```python
from build123d import *

# Parameters (mm, degrees)
SKETCH1_W = 17.5
SKETCH1_H = 8
FILLET1_R = 1


with BuildPart() as part:
    # Sketch1 → Revolve1 (revolve)
    with BuildSketch(Plane.XY, mode=Mode.PRIVATE) as revolve1_sk:
        with Locations((8.75, 4)):
            Rectangle(SKETCH1_W, SKETCH1_H)
    revolve(revolve1_sk.sketch.rotate(Axis((0, 0, 0), (0, 1, 0)), 90), axis=Axis((0, 0, 0), (0, 1, 0)))

    # Sketch2 → CSK for M3 Countersunk Flat Head Screw1 (revolve, cut)
    with BuildSketch(Plane(origin=(0, 8, 0), x_dir=(0, 0, 1), z_dir=(1, 0, 0))):
        Polygon((0, 0), (0, 8), (7.25, 8), (7.25, 5.25), (12.5, 0), align=None)
    revolve(axis=Axis((0, 14.35, 0), (0, -1, 0)), mode=Mode.SUBTRACT)

    # Fillet1
    fillet1_edges = [part.edges().sort_by_distance(p)[0] for p in [
        (0, 8, 17.5),
    ]]
    fillet(fillet1_edges, radius=FILLET1_R)


solid = part.part
```
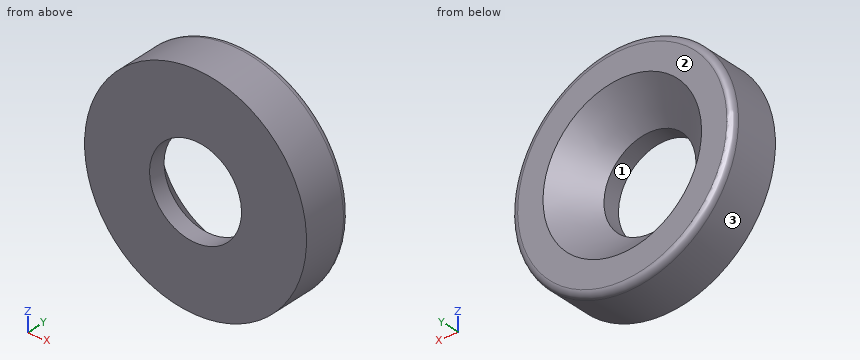
Work out the finished part from the listing and answer in its coordinate system (mm). Face numbers are marked on the shaded views. Give positions to 0.01 mm unless a question says otherwise; leave off trailing zeros. Order: outer loops, then holes, each group sorted by start corner. A loop starts at its lowest first (then second) coordinate and runs counter-clockwise, first axis right, second up. Notation, with made-up numbers: (55.25, -4) -> (97.25, -4) arc R34 ccw to (97.25, 33) -> close; hole circle Ø1 at (59.25, 81). An arc over 180 degrees is marked (long way). Answer as CSV lines item,"result". Start each with the question number.
(1) Section B-B, the plane z = 0 is taken. Write down the section's boundary in (x, y).
(2) Consider line 1 along X through (y, z) = (1.3, 0); line 2 along Z through (x, y) = (-6, 7.75); line 3 along Z through (x, y) = (-4.5, 7.5). Determine where each line is inside the solid, lowest interval first.
(3) Section C-C, the plane y = 6 is taken. Write down the section's boundary in (x, z), plus the area to 3 significant figures.
(4) Section D-D, the plane y = 4 is taken. Write down the section's boundary in (x, z).
(5) Section A-A, the plane x = 0 is taken. Write down the section's boundary in (y, z), plus the area to 3 significant figures.
(6) For a pull along X with two mould halves and no side action, classify the marked faces 1, 2 and 3 as released by +X, released by -X, zero draft, split by the parting line, or undercut.
(7) Each of these flat-tipped pins is pushed along its axis until it touches: pin 1 Ø3 at (x, y) = (5.5, 3) entering from +Z; pin 2 Ø2 at (y, z) = (3.5, -3.5) entering from -X; pin 3 Ø2 at (x, y) = (8, 2.5) entering from -Z. Where does it stop, or does it pass through?
Entries:
1,outline,"(-17.5, 0) -> (-7.25, 0) -> (-7.25, 2.75) -> (-12.5, 8) -> (-16.5, 8) arc R1 ccw to (-17.5, 7) -> close; (7.25, 0) -> (17.5, 0) -> (17.5, 7) arc R1 ccw to (16.5, 8) -> (12.5, 8) -> (7.25, 2.75) -> close"
2,line 1,"-17.5 to -7.25, 7.25 to 17.5"
2,line 2,"-16.08 to -10.68, 10.68 to 16.08"
2,line 3,"-16.77 to -11.12, 11.12 to 16.77"
3,outline,"circle Ø35 at (0, 0); hole circle Ø21 at (0, 0)"
3,area,"616 mm²"
4,outline,"circle Ø35 at (0, 0); hole circle Ø17 at (0, 0)"
5,outline,"(0, -17.5) -> (7, -17.5) arc R1 ccw to (8, -16.5) -> (8, -12.5) -> (2.75, -7.25) -> (0, -7.25) -> close; (0, 7.25) -> (2.75, 7.25) -> (8, 12.5) -> (8, 16.5) arc R1 ccw to (7, 17.5) -> (0, 17.5) -> close"
5,area,"136 mm²"
6,face 1,"undercut"
6,face 2,"zero draft"
6,face 3,"split by the parting line"
7,pin 1,"z = 17.04"
7,pin 2,"x = -17.32"
7,pin 3,"z = -16.04"
